from build123d import *

# Parameters (mm, degrees)
CYLINDER012_R     = 4.5
CYLINDER012_DEPTH = 10
CYLINDER011_R     = 5.5
CYLINDER011_DEPTH = 10
CYLINDER014_R     = 4.5
CYLINDER014_DEPTH = 10
CYLINDER013_R     = 5.5
CYLINDER013_DEPTH = 10
CYLINDER016_R     = 4.5
CYLINDER016_DEPTH = 10
CYLINDER015_R     = 5.5
CYLINDER015_DEPTH = 10
CYLINDER018_R     = 4.5
CYLINDER018_DEPTH = 10
CYLINDER017_R     = 5.5
CYLINDER017_DEPTH = 10
BOX023_W          = 10
BOX023_H          = 17
BOX023_DEPTH      = 1.75
CYLINDER010_R     = 1
CYLINDER010_DEPTH = 10
BOX022_W          = 14.5
BOX022_H          = 10
BOX022_DEPTH      = 6.5
FILLET009_R       = 0.5
BOX021_W          = 16.5
BOX021_H          = 10
BOX021_DEPTH      = 13.25
BOX020_W          = 9
BOX020_H          = 10
BOX020_DEPTH      = 3.17
FILLET008_R       = 1.2
BOX019_W          = 120
BOX019_H          = 120
BOX019_DEPTH      = 29.5
FILLET010_R       = 9
FILLET011_R       = 1


with BuildPart() as cylinder012:
    # Cylinder012 → Cylinder012 (new body)
    with BuildSketch(Plane(origin=(14.5, 14.5, -2.5), x_dir=(1, 0, 0), z_dir=(0, 0, 1))):
        Circle(CYLINDER012_R)
    extrude(amount=CYLINDER012_DEPTH)


with BuildPart() as base_pad001:
    # Cylinder011 → Cylinder011 (new body)
    with BuildSketch(Plane(origin=(14.5, 14.5, -2), x_dir=(1, 0, 0), z_dir=(0, 0, 1))):
        Circle(CYLINDER011_R)
    extrude(amount=CYLINDER011_DEPTH)

    # Fusion008: union Cylinder012
    add(cylinder012.part)


with BuildPart() as cylinder014:
    # Cylinder014 → Cylinder014 (new body)
    with BuildSketch(Plane(origin=(14.5, 14.5, -2.5), x_dir=(1, 0, 0), z_dir=(0, 0, 1))):
        Circle(CYLINDER014_R)
    extrude(amount=CYLINDER014_DEPTH)


with BuildPart() as base_pad002:
    # Cylinder013 → Cylinder013 (new body)
    with BuildSketch(Plane(origin=(14.5, 14.5, -2), x_dir=(1, 0, 0), z_dir=(0, 0, 1))):
        Circle(CYLINDER013_R)
    extrude(amount=CYLINDER013_DEPTH)

    # Fusion009: union Cylinder014
    add(cylinder014.part)


with BuildPart() as base_pad002_1:
    # Fusion009 placement: moved
    add(base_pad002.part.moved(Location((0, 89.5, 0))))


with BuildPart() as cylinder016:
    # Cylinder016 → Cylinder016 (new body)
    with BuildSketch(Plane(origin=(14.5, 14.5, -2.5), x_dir=(1, 0, 0), z_dir=(0, 0, 1))):
        Circle(CYLINDER016_R)
    extrude(amount=CYLINDER016_DEPTH)


with BuildPart() as base_pad003:
    # Cylinder015 → Cylinder015 (new body)
    with BuildSketch(Plane(origin=(14.5, 14.5, -2), x_dir=(1, 0, 0), z_dir=(0, 0, 1))):
        Circle(CYLINDER015_R)
    extrude(amount=CYLINDER015_DEPTH)

    # Fusion002: union Cylinder016
    add(cylinder016.part)


with BuildPart() as base_pad003_1:
    # Fusion002 placement: moved
    add(base_pad003.part.moved(Location((89.5, 0, 0))))


with BuildPart() as cylinder018:
    # Cylinder018 → Cylinder018 (new body)
    with BuildSketch(Plane(origin=(14.5, 14.5, -2.5), x_dir=(1, 0, 0), z_dir=(0, 0, 1))):
        Circle(CYLINDER018_R)
    extrude(amount=CYLINDER018_DEPTH)


with BuildPart() as base_pad004:
    # Cylinder017 → Cylinder017 (new body)
    with BuildSketch(Plane(origin=(14.5, 14.5, -2), x_dir=(1, 0, 0), z_dir=(0, 0, 1))):
        Circle(CYLINDER017_R)
    extrude(amount=CYLINDER017_DEPTH)

    # Fusion010: union Cylinder018
    add(cylinder018.part)


with BuildPart() as base_pad004_1:
    # Fusion010 placement: moved
    add(base_pad004.part.moved(Location((89.5, 89.5, 0))))


with BuildPart() as cube018:
    # Box023 → Box023 (new body)
    with BuildSketch(Plane(origin=(110, 76.5, 5.5), x_dir=(1, 0, 0), z_dir=(0, 0, 1))):
        with Locations((5, 8.5)):
            Rectangle(BOX023_W, BOX023_H)
    extrude(amount=BOX023_DEPTH)


with BuildPart() as cylinder010:
    # Cylinder010 → Cylinder010 (new body)
    with BuildSketch(Plane(origin=(92, 10, 10), x_dir=(1, 0, 0), z_dir=(0, -1, 0))):
        Circle(CYLINDER010_R)
    extrude(amount=CYLINDER010_DEPTH)


with BuildPart() as usb_hole:
    # Box022 → Box022 (new body)
    with BuildSketch(Plane.XY):
        with Locations((7.25, 5)):
            Rectangle(BOX022_W, BOX022_H)
    extrude(amount=BOX022_DEPTH)

    # Fillet009
    fillet009_edges = [usb_hole.edges().sort_by_distance(p)[0] for p in [
        (0, 5, 6.5),
        (0, 5, 0),
        (14.5, 5, 6.5),
        (14.5, 5, 0),
    ]]
    fillet(fillet009_edges, radius=FILLET009_R)


with BuildPart() as usb_hole_1:
    # Fillet009 placement: moved
    add(usb_hole.part.moved(Location((64.5, 0, 6.5))))


with BuildPart() as cube016:
    # Box021 → Box021 (new body)
    with BuildSketch(Plane(origin=(40.25, 0, 6), x_dir=(1, 0, 0), z_dir=(0, 0, 1))):
        with Locations((8.25, 5)):
            Rectangle(BOX021_W, BOX021_H)
    extrude(amount=BOX021_DEPTH)


with BuildPart() as fillet008:
    # Box020 → Box020 (new body)
    with BuildSketch(Plane(origin=(21.5, -6, 5.92), x_dir=(1, 0, 0), z_dir=(0, 0, 1))):
        with Locations((4.5, 5)):
            Rectangle(BOX020_W, BOX020_H)
    extrude(amount=BOX020_DEPTH)

    # Fillet008
    fillet008_edges = [fillet008.edges().sort_by_distance(p)[0] for p in [
        (21.5, -1, 9.09),
        (21.5, -1, 5.92),
        (30.5, -1, 9.09),
        (30.5, -1, 5.92),
    ]]
    fillet(fillet008_edges, radius=FILLET008_R)


with BuildPart() as fillet008_1:
    # Fillet008 placement: moved
    add(fillet008.part.moved(Location((0, 6, 0))))


with BuildPart() as gateway_box:
    # Box019 → Box019 (new body)
    with BuildSketch(Plane.XY):
        with Locations((60, 60)):
            Rectangle(BOX019_W, BOX019_H)
    extrude(amount=BOX019_DEPTH)

    # Cut012: cut Fillet008
    add(fillet008_1.part, mode=Mode.SUBTRACT)

    # Cut013: cut Cube016
    add(cube016.part, mode=Mode.SUBTRACT)

    # Cut014: cut USB_Hole
    add(usb_hole_1.part, mode=Mode.SUBTRACT)

    # Cut015: cut Cylinder010
    add(cylinder010.part, mode=Mode.SUBTRACT)

    # Cut016: cut Cube018
    add(cube018.part, mode=Mode.SUBTRACT)

    # Fillet010
    fillet010_edges = [gateway_box.edges().sort_by_distance(p)[0] for p in [
        (0, 0, 14.75),
        (0, 120, 14.75),
        (120, 0, 14.75),
        (120, 120, 14.75),
    ]]
    fillet(fillet010_edges, radius=FILLET010_R)

    # Fusion004: union base_pad001, base_pad002, base_pad003, base_pad004
    add(base_pad001.part)
    add(base_pad002_1.part)
    add(base_pad003_1.part)
    add(base_pad004_1.part)

    # Fillet011
    fillet011_edges = [gateway_box.edges().sort_by_distance(p)[0] for p in [
        (0, 60, 29.5),
        (0, 111, 14.75),
        (2.636039, 2.636039, 29.5),
        (2.636039, 117.363961, 29.5),
        (60, 0, 29.5),
        (60, 120, 29.5),
        (117.363961, 2.636039, 29.5),
        (117.363961, 117.363961, 29.5),
        (120, 60, 29.5),
        (2.636039, 2.636039, 0),
        (2.636039, 117.363961, 0),
        (9, 120, 14.75),
        (60, 0, 0),
        (60, 120, 0),
        (117.363961, 2.636039, 0),
        (117.363961, 117.363961, 0),
    ]]
    fillet(fillet011_edges, radius=FILLET011_R)


solid = gateway_box.part
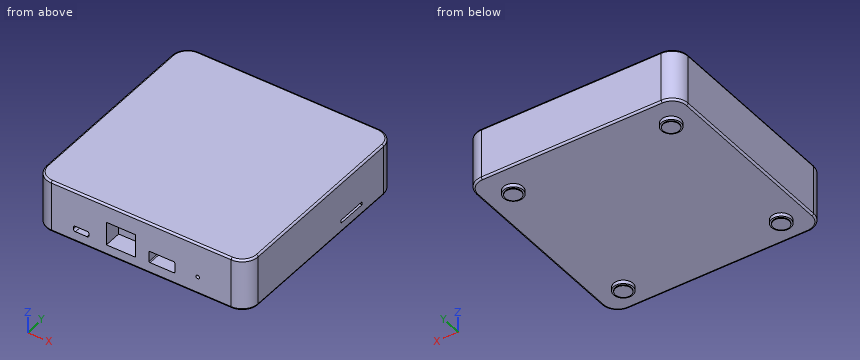
The listing builds one solid part. Answer for the finished solid, in the listing's coordinates (mm). Coordinates: 2 decimals unless noted, no trailing zeros. Loops run counter-clockwise (first coordinate to the right, second up) from the corner with the lowest first, then second, coordinate; pieces in that order, holes last.
1) Find section C-C on x = 104. Write down the section's boundary in (y, z).
2) Flat-ended cylindrical pins translate along their axes: pin 1 Ø10 at (x, y) = (28, 92.5) entering from -Z; pin 2 Ø0.6 at (x, z) = (92, 9.5) entering from -Y; pin 3 Ø1.9 at (x, z) = (115.5, 6.5) entering from +Y. Find the tip coordinate at first contact, or state that the pin passes through.
3) Find section A-A on x = 87. Write down the section's boundary in (y, z).
4) Find the intervals of material crossed by L1, parallel to Z at x = 92, y = 2; L2, parallel to Z at x = 52.5, y = 49.5; L3, parallel to Y at x = 8.5, z = 17.5, in increasing order.
Values:
1. outline: (0, 1) arc R1 ccw to (1, 0) - (9, 0) - (9, -2) - (10, -2) - (10, -2.5) - (19, -2.5) - (19, -2) - (20, -2) - (20, 0) - (98.5, 0) - (98.5, -2) - (99.5, -2) - (99.5, -2.5) - (108.5, -2.5) - (108.5, -2) - (109.5, -2) - (109.5, 0) - (119, 0) arc R1 ccw to (120, 1) - (120, 28.5) arc R1 ccw to (119, 29.5) - (1, 29.5) arc R1 ccw to (0, 28.5) - close
2. pin 1: stops at z = 0
2. pin 2: stops at y = 10
2. pin 3: stops at y = 119.27
3. outline: (0, 1) arc R1 ccw to (1, 0) - (119, 0) arc R1 ccw to (120, 1) - (120, 28.5) arc R1 ccw to (119, 29.5) - (1, 29.5) arc R1 ccw to (0, 28.5) - close
4. L1: z = 0 to 9, 11 to 29.5
4. L2: z = 0 to 29.5
4. L3: y = 0.01 to 119.99
